Check sheet for the drawn part. Datum: minimum x, y, z corner. Units: mm. Give positions to 0.01 mm unless a question says otherwise; leave off trailing zeros. Order: outer loops, then holes, each group sorted by start corner. A loop starts at its lowest first (then second) coordinate and runs counter-clockwise, first axis right, second up.
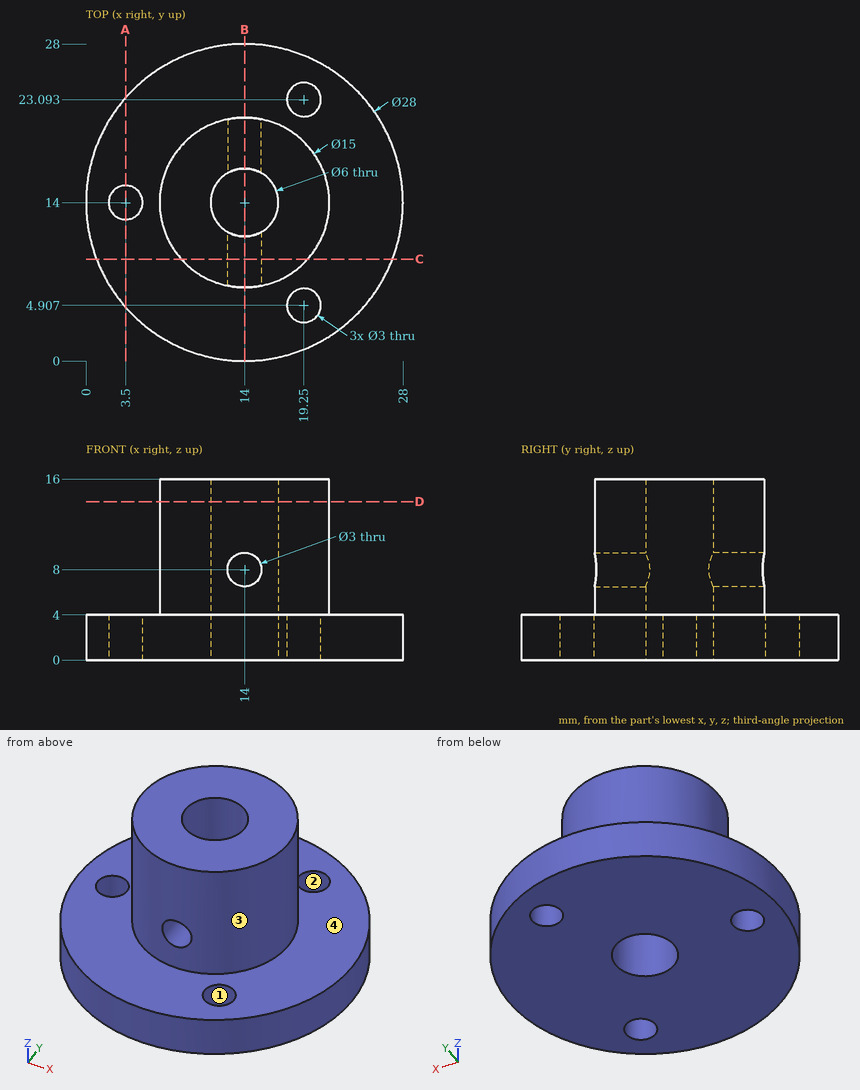
(1) Release check for a two-part mould opening along X. For the marked faces 1, 2, 3 and 4 record: pulls with the +X half, pulls with the -X half, needs draft (parallel to the pull), parting line crosses it, or undercut.
Solved:
face 1: undercut
face 2: undercut
face 3: parting line crosses it
face 4: needs draft
(2) Section check A-A, the plane x = 3.5. Enter the section's corners in (y, z).
Solved:
outline: (4.74, 0) - (12.5, 0) - (12.5, 4) - (4.74, 4) - close; (15.5, 0) - (23.26, 0) - (23.26, 4) - (15.5, 4) - close
(3) Section check B-B, the plane x = 14. Enter the section's corners in (y, z).
Solved:
outline: (0, 0) - (11, 0) - (11, 6.5) - (6.5, 6.5) - (6.5, 4) - (0, 4) - close; (6.5, 9.5) - (11, 9.5) - (11, 16) - (6.5, 16) - close; (17, 0) - (28, 0) - (28, 4) - (21.5, 4) - (21.5, 6.5) - (17, 6.5) - close; (17, 9.5) - (21.5, 9.5) - (21.5, 16) - (17, 16) - close
(4) Section check D-D, the plane z = 14. Enter the section's corners in (x, y), then the cut area to 3 significant figures.
Solved:
outline: circle Ø15 at (14, 14); hole circle Ø6 at (14, 14)
area: 148 mm2
(5) Section check C-C, the plane y = 9. Enter the section's corners in (x, z), then the cut area to 3 significant figures.
Solved:
outline: (0.92, 0) - (27.08, 0) - (27.08, 4) - (19.59, 4) - (19.59, 16) - (8.41, 16) - (8.41, 4) - (0.92, 4) - close; hole circle Ø3 at (14, 8)
area: 232 mm2
(6) Scan lines: line 1 (Y direction, x = 19.25, z = 2.5); line 2 (Z direction, x = 4.5, y = 5.25); line 3 (Y direction, x = 3.5, z = 1.7). Record each from-to range of solid material in increasing order.
Solved:
line 1: y = 1.02 to 3.41, 6.41 to 21.59, 24.59 to 26.98
line 2: z = 0 to 4
line 3: y = 4.74 to 12.5, 15.5 to 23.26
(7) Go/stop test with flat-tipped pins: pin 1 (5 mm diameter, centred on y = 11, z = 13.5, fed in from -X); pin 2 (5 mm diameter, centred on x = 25, y = 3.5, fed in from +Z); pin 3 (6 mm diameter, centred on x = 15, z = 11.5, fed in from -Y). Record where each tip stops, or that it passes through.
Solved:
pin 1: stops at x = 6.52
pin 2: stops at z = 4
pin 3: stops at y = 6.5
